Input: part model. Units: mm. Frame: model coordinates. Give positions to 0.01 mm unless a question says otherwise; leave off trailing zeros. Order: outer loops, then holes, each group sorted by start corner. A loop starts at its lowest first (then second) coordinate and runs counter-clockwise, first axis right, second up. Notation, with made-up numbers: (39, 8) - (77, 8) arc R32 ccw to (77, 42) - close; hole circle Ø5 at (48, -17.5). An arc over 180 degrees is marked (long way). Answer in a Markdown table with one row per item. Add a question column.
1. Contact query for flat-ended pins moving along their axis: pin 1 (2 mm diameter, centred on x = 41.5, z = 56.5, fed in from +Y); pin 2 (10 mm diameter, centred on x = 61, z = 55.5, fed in from +Y). Output: stop coordinate, or through.
2. Section query C-C on z = 64.5. Return loops of the section in (x, y), and give its area (3 significant figures).
3. Section query B-B on y = 84. Return loops of the section in (x, z).
4. Section query A-A on x = 68. Return loops of the section in (y, z).
5. Ray query, line 1 (Y direction, x = 73, z = 39); line 2 (Z direction, x = 31.5, y = 6.5); line 3 (Z direction, x = 29, y = 27). Return the intervals inside material, ascending. Write a range as [from, to].
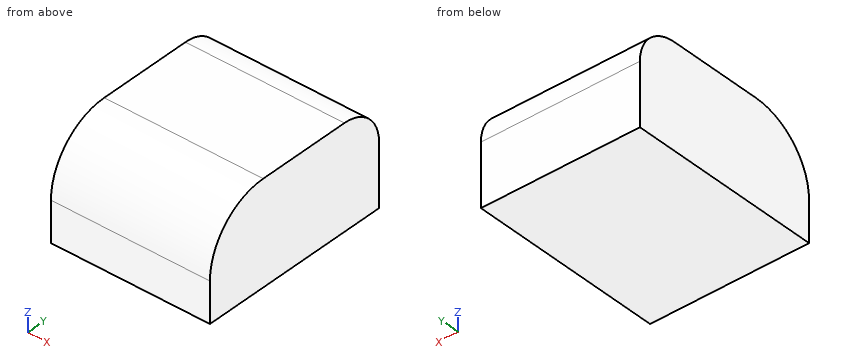
```python
from build123d import *

# Parameters (mm, degrees)
F0_W     = 75.997784
F0_H     = 48.82941
F1_DEPTH = 93.811005
F2_R     = 19.21578
F3_R     = 29.563082


with BuildPart() as f1:
    # F0 (on Front) → F1 (new body)
    with BuildSketch(Plane.XZ):
        with Locations((46.23688, 43.56139)):
            Rectangle(F0_W, F0_H)
    extrude(amount=-F1_DEPTH)

    # F2
    f2_edges = [f1.edges().sort_by_distance(p)[0] for p in [
        (46.23688, 93.811005, 67.976095),
    ]]
    fillet(f2_edges, radius=F2_R)

    # F3
    f3_edges = [f1.edges().sort_by_distance(p)[0] for p in [
        (46.23688, 0, 67.976095),
    ]]
    fillet(f3_edges, radius=F3_R)


solid = f1.part
```
Answer:
| question | item | result |
|---|---|---|
| 1 | pin 1 | stops at y = 92.59 |
| 1 | pin 2 | stops at y = 93.73 |
| 2 | outline | (8.24, 15.65) - (84.24, 15.65) - (84.24, 85.62) - (8.24, 85.62) - close |
| 2 | area | 5,320 mm² |
| 3 | outline | (8.24, 19.15) - (84.24, 19.15) - (84.24, 65.52) - (8.24, 65.52) - close |
| 4 | outline | (0, 19.15) - (93.81, 19.15) - (93.81, 48.76) arc R19.22 ccw to (74.6, 67.98) - (29.56, 67.98) arc R29.56 ccw to (0, 38.41) - close |
| 5 | line 1 | y = [0.01, 93.81] |
| 5 | line 2 | z = [19.15, 56.91] |
| 5 | line 3 | z = [19.15, 67.86] |
